```python
from build123d import *

# Parameters (mm, degrees)
SKETCH2_W           = 81
SKETCH2_H           = 81
BOSS_EXTRUDE1_DEPTH = 10


with BuildPart() as part:
    # Sketch1 → Revolve1 (revolve)
    with BuildSketch(Plane.XY):
        with BuildLine():
            Line((0, 10), (0, 0))
            Line((0, 0), (30.5, 0))
            add(Edge.make_bspline(
                [(30.5, 0), (24.462439427, 10.588096747), (11.157200838, 9.492825223), (0, 10)],
                knots=[0, 0, 0, 0, 1, 1, 1, 1], degree=3))
        make_face()
    revolve(axis=Axis((0, 10, 0), (0, -1, 0)))

    # Sketch2 → Boss-Extrude1 (add)
    with BuildSketch(Plane(origin=(0, 0, 0), x_dir=(1, 0, 0), z_dir=(0, 1, 0))):
        Rectangle(SKETCH2_W, SKETCH2_H)
    extrude(amount=-BOSS_EXTRUDE1_DEPTH)


solid = part.part
```
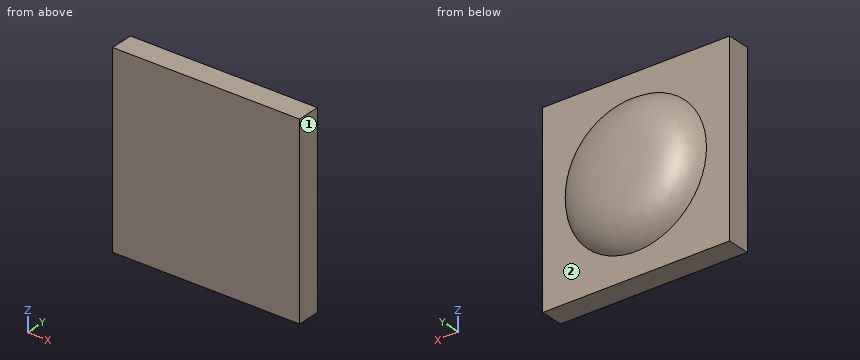
Work out the finished part from the listing and answer in its coordinate system (mm). Face numbers are marked on the shaded views. A direction names the side the tool comes from. Give positions to 0.01 mm unless a question says otherwise; leave off trailing zeros. Write each loop counter-clockwise with the first axis right and the second up, starting at its lowest first coordinate (ties: lowest second). Pieces come first, ordered by that corner, then holes.
(1) The part is cut by section B-B on x = 33. Write down the section's boundary in (y, z).
Final values:
outline: (-10, -40.5) - (0, -40.5) - (0, 40.5) - (-10, 40.5) - close
(2) Straight lines are drawn through the part: line 1 (Y direction, x = -25.5, z = 36); line 2 (Y direction, x = -26.5, z = 10.5); line 3 (Z direction, x = -7, y = 3.25). For each, find the intervals that lie inside material, in ascending order.
Final values:
line 1: y = -10 to 0
line 2: y = -10 to 2.81
line 3: z = -27.22 to 27.22
(3) Flat-ended cylindrical pins translate along their axes: pin 1 Ø1.5 at (x, z) = (-15, -27) entering from +Y; pin 2 Ø5 at (x, z) = (1, 22) entering from +Y; pin 3 Ø4 at (x, y) = (20.5, 3.5) entering from -Z. Find the tip coordinate at first contact, or state that the pin passes through.
Final values:
pin 1: stops at y = 0.61
pin 2: stops at y = 8.21
pin 3: stops at z = -21.98
(4) The part is cut by section A-A on z = 35. Write down the section's boundary in (x, y).
Final values:
outline: (-40.5, -10) - (40.5, -10) - (40.5, 0) - (-40.5, 0) - close
(5) Which of the six approach directions +Z, -Z, +X, -X, +Y, -Y give full straight-line access (tool end or side, diameter ignored) to the marked faces 1 and 2?
Final values:
face 1: +Z, -Z, +X, +Y, -Y
face 2: +Y
